Read the model definition and answer for the solid it produces. Units are mm, in the model's axes. Face numbers are marked on the shaded views. A direction names the side the tool comes from. Give positions to 0.01 mm unless a question says otherwise; leave off trailing zeros. Order: outer loops, then holes, each group sorted by start corner. A loop starts at its lowest first (then second) coordinate and runs counter-clockwise, first axis right, second up. Notation, with made-up numbers: M 6,33.25 L 13,33.25 A20 cw 13,70.25 Z; hole C 36.25,-10 d5. An arc over 180 degrees is marked long. One line per item, written item: value.
from build123d import *

# Parameters (mm, degrees)
SKETCH1_R           = 27.5
BOSS_EXTRUDE1_DEPTH = 16
CUT_EXTRUDE1_DEPTH  = 15
CUT_EXTRUDE2_DEPTH  = 15
SKETCH6_W           = 18.849176954
SKETCH6_H           = 19.96776686
CUT_EXTRUDE4_DEPTH  = 10
CHAMFER2_SIZE       = 3
CHAMFER3_SIZE       = 3
SKETCH8_W           = 7.009579852
SKETCH8_H           = 10.026822324
CUT_EXTRUDE5_DEPTH  = 15
CHAMFER4_SIZE       = 1
CHAMFER5_SIZE       = 2
CHAMFER6_SIZE       = 2
CHAMFER7_SIZE       = 1
CHAMFER8_SIZE       = 0.5
SKETCH9_W           = 10.5
SKETCH9_H           = 5.1
CUT_EXTRUDE6_DEPTH  = 5.5


with BuildPart() as part:
    # Sketch1 → Boss-Extrude1 (new body)
    with BuildSketch(Plane(origin=(0, 0, 0), x_dir=(1, 0, 0), z_dir=(0, 1, 0))):
        Circle(SKETCH1_R)
    extrude(amount=BOSS_EXTRUDE1_DEPTH)

    # Sketch3 → Cut-Extrude1 (cut)
    with BuildSketch(Plane(origin=(0, 16, 0), x_dir=(1, 0, 0), z_dir=(0, 1, 0))):
        Polygon((-11.25, -16.25), (16.25, -16.25), (21.25, -16.25), (21.25, 16.25), (16.25, 16.25), (-11.25, 16.25), align=None)
    extrude(amount=-CUT_EXTRUDE1_DEPTH, mode=Mode.SUBTRACT)

    # Sketch4 → Cut-Extrude2 (cut)
    with BuildSketch(Plane.ZY.offset(-21.25)):
        with BuildLine():
            Line((-2.103243144, 13.902406248), (2.103243144, 13.902406248))
            ThreePointArc((2.103243144, 13.902406248), (0, 6.5), (-2.103243144, 13.902406248))
        make_face()
    extrude(amount=-CUT_EXTRUDE2_DEPTH, mode=Mode.SUBTRACT)

    # Sketch6 → Cut-Extrude4 (cut)
    with BuildSketch(Plane(origin=(0, 16, 0), x_dir=(1, 0, 0), z_dir=(0, 1, 0))):
        with Locations((-11.25, 0)):
            Rectangle(SKETCH6_W, SKETCH6_H)
    extrude(amount=-CUT_EXTRUDE4_DEPTH, mode=Mode.SUBTRACT)

    # Chamfer2
    chamfer2_edges = [part.edges().sort_by_distance(p)[0] for p in [
        (-11.25, 6, 0),
        (-11.25, 11, -9.98388343),
        (-11.25, 11, 9.98388343),
        (-15.962294239, 6, 9.98388343),
        (-15.962294239, 6, -9.98388343),
        (-20.674588477, 6, 0),
    ]]
    chamfer(chamfer2_edges, length=CHAMFER2_SIZE)

    # Chamfer3
    chamfer3_edges = [part.edges().sort_by_distance(p)[0] for p in [
        (-20.674588477, 12.5, 9.98388343),
        (-20.674588477, 12.5, -9.98388343),
    ]]
    chamfer(chamfer3_edges, length=CHAMFER3_SIZE)

    # Sketch8 → Cut-Extrude5 (cut)
    with BuildSketch(Plane(origin=(0, 16, 0), x_dir=(1, 0, 0), z_dir=(0, 1, 0))):
        with Locations((21.25, 0)):
            Rectangle(SKETCH8_W, SKETCH8_H)
    extrude(amount=-CUT_EXTRUDE5_DEPTH, mode=Mode.SUBTRACT)

    # Chamfer4
    chamfer4_edges = [part.edges().sort_by_distance(p)[0] for p in [
        (24.754789926, 6.5, 0),
        (24.754789926, 13.902406248, 0),
    ]]
    chamfer(chamfer4_edges, length=CHAMFER4_SIZE)

    # Chamfer5
    chamfer5_edges = [part.edges().sort_by_distance(p)[0] for p in [
        (24.754789926, 1, 0),
    ]]
    chamfer(chamfer5_edges, length=CHAMFER5_SIZE)

    # Chamfer6
    chamfer6_edges = [part.edges().sort_by_distance(p)[0] for p in [
        (-11.25, 16, -14.616941715),
        (-11.25, 16, 14.616941715),
    ]]
    chamfer(chamfer6_edges, length=CHAMFER6_SIZE)

    # Chamfer7
    chamfer7_edges = [part.edges().sort_by_distance(p)[0] for p in [
        (22.002394963, 1, 5.013411162),
        (22.002394963, 1, -5.013411162),
        (5, 1, -16.25),
        (21.25, 1, 10.631705581),
        (5, 1, 16.25),
        (-11.25, 1, 0),
        (21.25, 1, -10.631705581),
    ]]
    chamfer(chamfer7_edges, length=CHAMFER7_SIZE)

    # Chamfer8
    chamfer8_edges = [part.edges().sort_by_distance(p)[0] for p in [
        (27.479855714, 13.902406248, 1.05239247),
    ]]
    chamfer(chamfer8_edges, length=CHAMFER8_SIZE)

    # Sketch9 → Cut-Extrude6 (cut)
    with BuildSketch(Plane(origin=(0, 16, 0), x_dir=(1, 0, 0), z_dir=(0, 1, 0))):
        with Locations((0, 21.833387082)):
            Rectangle(SKETCH9_W, SKETCH9_H)
        with Locations((0, -21.833387082)):
            Rectangle(SKETCH9_W, SKETCH9_H)
    extrude(amount=-CUT_EXTRUDE6_DEPTH, mode=Mode.SUBTRACT)


solid = part.part
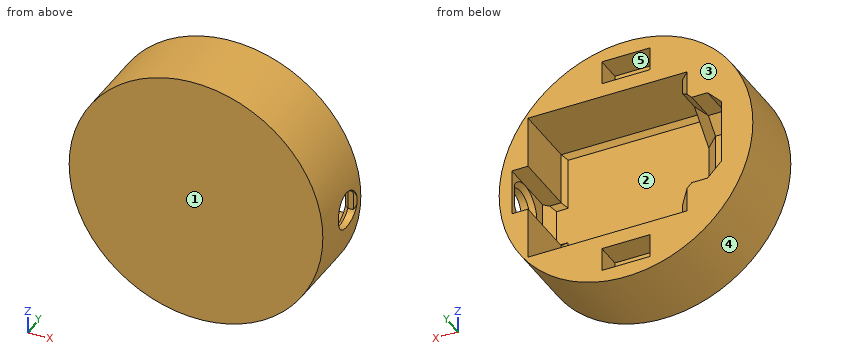
1) Each of these flat-tipped pins is pushed along its axis until it touches: pin 1 Ø4 at (x, z) = (-1.5, 22) entering from +Y; pin 2 Ø3 at (x, y) = (-1.5, 14) entering from +Z; pin 3 Ø1.5 at (y, z) = (3.5, 12.5) entering from +X; pin 4 Ø6 at (x, z) = (-12.5, -6) entering from -Y. Where does it stop, or does it pass through?
Reported:
pin 1: stops at y = 10.5
pin 2: stops at z = 27.5
pin 3: stops at x = 24.86
pin 4: stops at y = 0
2) Find section C-C, the plane y = 4.75. Write down the section's boundary in (x, z), plus the area to 3 significant figures.
Reported:
outline: C 0,0 d55; hole M -13,-6.98 L -11.25,-8.73 L -11.25,-16.25 L 21.25,-16.25 L 21.25,-5.01 L 24.75,-5.01 L 24.75,5.01 L 21.25,5.01 L 21.25,16.25 L -11.25,16.25 L -11.25,8.73 L -13,6.98 Z
area: 1,260 mm^2
3) Find section D-D, the plane y = 12.5. Count the separate pieces of the cut face and the enclosed holes in it, plus the area to 3 significant figures.
Reported:
separate pieces: 1
enclosed holes: 2
area: 970 mm^2
4) Find section A-A, the plane z = 0. Write down the section's boundary in (x, y).
Reported:
outline: M -27.5,0 L 27.5,0 L 27.5,6.5 L 25.75,6.5 L 24.75,5.5 L 24.75,3 L 22.75,1 L -10.25,1 L -11.25,2 L -11.25,3 L -14.25,6 L -17.67,6 L -20.67,9 L -20.67,16 L -27.5,16 Z; M 24.75,14.9 L 25.75,13.9 L 27,13.9 L 27.5,14.4 L 27.5,16 L 24.75,16 Z
5) Which of the six approach directions +Z, -Z, +X, -X, +Y, -Y give full straight-line access (tool end or side, diameter ignored) to the marked faces 1 and 2?
Reported:
face 1: +Z, -Z, +X, -X, -Y
face 2: +Y
6) Determine the mould class of the marked faces 3, 4 and 5 for opening direction Z: +Z half, -Z half, draft (parallel to the pull), parting line (faces both ways), or undercut.
Reported:
face 3: draft
face 4: parting line
face 5: undercut
7) Consider probe 1 along Y at (x, z) = (26.85, 0); probe 2 along Z at (x, y) = (2.5, 15.75); probe 3 along Z at (x, y) = (-16.5, 9.25). Determine where each line is inside the solid, lowest interval first.
Reported:
probe 1: y = 0 to 6.5, 13.9 to 16
probe 2: z = -27.39 to -24.38, -19.28 to -16.25, 16.25 to 19.28, 24.38 to 27.39
probe 3: z = -22 to -9.98, 9.98 to 22
8) Find section B-B, the plane x = 0. Write down the section's boundary in (y, z).
Reported:
outline: M 0,-27.5 L 16,-27.5 L 16,-24.38 L 10.5,-24.38 L 10.5,-19.28 L 16,-19.28 L 16,-16.25 L 2,-16.25 L 1,-15.25 L 1,15.25 L 2,16.25 L 16,16.25 L 16,19.28 L 10.5,19.28 L 10.5,24.38 L 16,24.38 L 16,27.5 L 0,27.5 Z
